```python
from build123d import *

# Parameters (mm, degrees)
PAD001_DEPTH                = 1
BOX_W                       = 1
BOX_H                       = 4
BOX_DEPTH                   = 62
BOX_PLACEMENT_ANGLE         = 340
CYLINDER_R                  = 2
CYLINDER_DEPTH              = 67
CYLINDER_PLACEMENT_ANGLE    = 340
CYLINDER001_R               = 4
CYLINDER001_DEPTH           = 60
CYLINDER001_PLACEMENT_ANGLE = 20
SKETCH_R                    = 2.527902
PAD_DEPTH                   = 10
FILLET_R                    = 2
FILLET001_R                 = 2
FILLET003_R                 = 1


with BuildPart() as body001:
    # Sketch001 → Pad001 (new body, symmetric)
    with BuildSketch(Plane.YZ):
        Polygon((11.126045, 25.12734), (5.15667, 9.780665), (10.086619, 0), (14.214679, 32.616486), align=None)
    extrude(amount=PAD001_DEPTH, both=True)


with BuildPart() as box:
    # Box → Box (new body)
    with BuildSketch(Plane.XY):
        with Locations((0.5, 2)):
            Rectangle(BOX_W, BOX_H)
    extrude(amount=BOX_DEPTH)


with BuildPart() as box_1:
    # Box placement: moved
    add(box.part.moved(Location((0, -5.296136, 2.991813))).rotate(Axis((0, -5.296136, 2.991813), (1, 0, 0)), BOX_PLACEMENT_ANGLE))


with BuildPart() as cylinder:
    # Cylinder → Cylinder (new body)
    with BuildSketch(Plane.XY):
        Circle(CYLINDER_R)
    extrude(amount=CYLINDER_DEPTH)


with BuildPart() as cylinder_1:
    # Cylinder placement: moved
    add(cylinder.part.moved(Location((0, -2.318081, -1.61877))).rotate(Axis((0, -2.318081, -1.61877), (1, 0, 0)), CYLINDER_PLACEMENT_ANGLE))


with BuildPart() as cylinder001:
    # Cylinder001 → Cylinder001 (new body)
    with BuildSketch(Plane.XY):
        Circle(CYLINDER001_R)
    extrude(amount=CYLINDER001_DEPTH)


with BuildPart() as cylinder001_1:
    # Cylinder001 placement: moved
    add(cylinder001.part.moved(Location((0, -0.95, 2.14))).rotate(Axis((0, -0.95, 2.14), (-1, 0, 0)), CYLINDER001_PLACEMENT_ANGLE))


with BuildPart() as fillet003:
    # Sketch → Pad (new body)
    with BuildSketch(Plane.XY):
        with BuildLine():
            ThreePointArc((-11.024148, 4.03498), (-16.038919, -1.856194), (-8.310522, -1.501592))
            Line((-8.310522, -1.501592), (0, -1.501592))
            Line((8.310522, -1.501592), (0, -1.501592))
            ThreePointArc((8.310522, -1.501592), (16.038919, -1.856194), (11.024148, 4.03498))
            Line((11.024148, 4.03498), (3.534046, 10.276075))
            Line((3.534046, 10.276075), (0, 10.276075))
            Line((-3.534046, 10.276075), (0, 10.276075))
            Line((-11.024148, 4.03498), (-3.534046, 10.276075))
        make_face()
        with Locations((-12.251753, 0)):
            Circle(SKETCH_R, mode=Mode.SUBTRACT)
        with Locations((12.251753, 0)):
            Circle(SKETCH_R, mode=Mode.SUBTRACT)
    extrude(amount=PAD_DEPTH)

    # Fusion: union Cylinder001
    add(cylinder001_1.part)

    # Cut: cut Cylinder
    add(cylinder_1.part, mode=Mode.SUBTRACT)

    # Cut001: cut Box
    add(box_1.part, mode=Mode.SUBTRACT)

    # Fillet
    fillet_edges = [fillet003.edges().sort_by_distance(p)[0] for p in [
        (-1.866147, 5.675875, 10),
    ]]
    fillet(fillet_edges, radius=FILLET_R)

    # Fusion001: union Body001
    add(body001.part)

    # Fillet001
    fillet001_edges = [fillet003.edges().sort_by_distance(p)[0] for p in [
        (-3.534046, 10.276075, 5),
    ]]
    fillet(fillet001_edges, radius=FILLET001_R)

    # Fillet003
    fillet003_edges = [fillet003.edges().sort_by_distance(p)[0] for p in [
        (-7.557221, 6.923782, 10),
        (7.279097, 7.155528, 10),
    ]]
    fillet(fillet003_edges, radius=FILLET003_R)


solid = fillet003.part
```
Here's how the part is built. I have some questions about the finished solid (model axes, mm). A direction names the side the tool comes from. Give positions to 0.01 mm unless a question says otherwise; leave off trailing zeros. Loops run counter-clockwise (first coordinate to the right, second up) from the corner with the lowest first, then second, coordinate; pieces in that order, holes last. Notation, with made-up numbers: M 9,26.25 L 63,26.25 A32 ccw 63,61.25 Z; hole C 80.25,39 d4. An arc over 180 degrees is marked long. Use one line per item in the form item = value. Start each with the question number.
Q1. Which directions (+Z, -Z, +X, -X, +Y, -Y) give clear straight access to the entire face, cutting with the end or side of a thin tool? Please do faces 1 (the flat face through (2, 10.276, 5)), 2 (the flat face through (2, 21, 58)), 3 (the flat face through (2.13, -2.68, 2.77)), 4 (the flat face through (1, 7, 31)), 5 (the flat face through (0, 3, 0)).
Q2. Thinking about a two-plate mould opening in Y: for faces 6 (the cylindrical face through (-14.777, 0.111, 4.93)), 7 (the flat face through (0, 12.2, 16.7)), 8 (the cylindrical face through (-0.44, 10.62, 28.22)), 9 (the cylindrical face through (-1.47, 7.95, 37.47)), which applies, +Y half, -Y half, draft (parallel to the pull), parting line (faces both ways), or undercut?
Q3. If we section it at A-A (x = -12): Write out the boundary of the cut face in (y, z), then the cut area to 3 significant figures.
Q4. I need wall thicknesses on line 1 along Z through (x, y) = (-7, 6.25); line 2 along Y through (x, z) = (-10, 9); line 3 along X through (y, z) = (11.25, 31). Which ranges of each line are inside material? Lowest first, please.
Q5. Will these pins go through, and if not, where does the flat tip stop? pin 1 Ø1 at (x, z) = (1, 33.5) entering from +Y; pin 2 Ø8 at (y, z) = (14, 24) entering from -X; pin 3 Ø8 at (y, z) = (12, 12) entering from -X; pin 4 Ø1.5 at (y, z) = (13.5, 15) entering from +X.
Q6. If we section it at B-B (y = 0): State how many separate pieces and enclosed holes the cut face has, then the cut area to 3 significant figures.
Taken from the geometry:
q1.face_1 = -Z, +Y
q1.face_2 = +Z, +X, -X, +Y
q1.face_3 = -Z, -Y
q1.face_4 = +Z, -Y
q1.face_5 = -Z, +X, -X, +Y, -Y
q2.face_6 = undercut
q2.face_7 = +Y half
q2.face_8 = undercut
q2.face_9 = parting line
q3.outline = M -4.21,0 L -2.52,0 L -2.52,10 L -4.21,10 Z; M 2.52,0 L 4.21,0 L 4.21,10 L 2.52,10 Z
q3.area = 33.9 mm^2
q4.line_1 = 0 to 9.99
q4.line_2 = -3.57 to -1.15, 1.15 to 4.89
q4.line_3 = -3.67 to -1.21, 1.21 to 3.67
q5.pin_1 = 14.8
q5.pin_2 = -3.06
q5.pin_3 = -5
q5.pin_4 = through
q6.separate_pieces = 4
q6.enclosed_holes = 0
q6.area = 221 mm^2
